Geometry check sheet. Reference: the model listing, model coordinates, mm. Face numbers are marked on the shaded views. A direction names the side the tool comes from. Coordinates: 2 decimals unless noted, no trailing zeros. Loops run counter-clockwise (first coordinate to the right, second up) from the corner with the lowest first, then second, coordinate; pieces in that order, holes last. Notation, with made-up numbers: M 52.25,23 L 89.25,23 A20 ccw 89.25,48 Z; hole C -3.5,57 d10. An arc over 180 degrees is marked long. One line per question, with ' | ' between items. Start each with the question number.
from build123d import *

# Parameters (mm, degrees)
M42_CLEARANCE_HOLE1_D                           = 47
M42_CLEARANCE_HOLE1_DEPTH                       = 4.5
SKETCH4_W                                       = 7
SKETCH4_H                                       = 4.5
CSK_FOR_M2_FLAT_HEAD_MACHINE_SCREW1_D           = 2.2
CSK_FOR_M2_FLAT_HEAD_MACHINE_SCREW1_DEPTH       = 6
CSK_FOR_M2_FLAT_HEAD_MACHINE_SCREW1_CSINK_D     = 4.4
CSK_FOR_M2_FLAT_HEAD_MACHINE_SCREW1_CSINK_ANGLE = 90
CBORE_FOR_M8_HEX_HEAD_BOLT1_D                   = 10
CBORE_FOR_M8_HEX_HEAD_BOLT1_DEPTH               = 6
CBORE_FOR_M8_HEX_HEAD_BOLT1_CBORE_D             = 11.2
CBORE_FOR_M8_HEX_HEAD_BOLT1_CBORE_DEPTH         = 1.2


with BuildPart() as part:
    # Sketch1 → Revolve1 (revolve)
    with BuildSketch(Plane(origin=(0, 0, 0), x_dir=(1, 0, 0), z_dir=(0, 1, 0))):
        Polygon((25.5, 0), (0, 0), (0, -6), (25.5, -6), (25.5, -5.5), (25, -5.5), (25, -0.5), (25.5, -0.5), align=None)
    revolve(axis=Axis((0, 0, 0), (0, 0, 1)))

    # M42 Clearance Hole1
    with Locations(Plane.XY.offset(6)):
        with Locations((0, 0)):
            Hole(M42_CLEARANCE_HOLE1_D / 2, depth=M42_CLEARANCE_HOLE1_DEPTH)

    # Sketch4 → Revolve2 (revolve)
    with BuildSketch(Plane(origin=(0, 0, 0), x_dir=(1, 0, 0), z_dir=(0, 1, 0))):
        with Locations((3.5, -3.75)):
            Rectangle(SKETCH4_W, SKETCH4_H)
    revolve(axis=Axis((0, 0, 1.5), (0, 0, 1)))

    # CSK for M2 Flat Head Machine Screw1
    with Locations(Plane(origin=(0, 0, 0), x_dir=(-1, 0, 0), z_dir=(0, 0, -1))):
        with Locations((-7.794228634, -4.5), (7.794228634, -4.5), (0, 9)):
            CounterSinkHole(CSK_FOR_M2_FLAT_HEAD_MACHINE_SCREW1_D / 2, CSK_FOR_M2_FLAT_HEAD_MACHINE_SCREW1_CSINK_D / 2, depth=CSK_FOR_M2_FLAT_HEAD_MACHINE_SCREW1_DEPTH, counter_sink_angle=CSK_FOR_M2_FLAT_HEAD_MACHINE_SCREW1_CSINK_ANGLE)

    # CBORE for M8 Hex Head Bolt1
    with Locations(Plane(origin=(0, 0, 0), x_dir=(-1, 0, 0), z_dir=(0, 0, -1))):
        with Locations((0, 0)):
            CounterBoreHole(CBORE_FOR_M8_HEX_HEAD_BOLT1_D / 2, CBORE_FOR_M8_HEX_HEAD_BOLT1_CBORE_D / 2, CBORE_FOR_M8_HEX_HEAD_BOLT1_CBORE_DEPTH, depth=CBORE_FOR_M8_HEX_HEAD_BOLT1_DEPTH)


solid = part.part
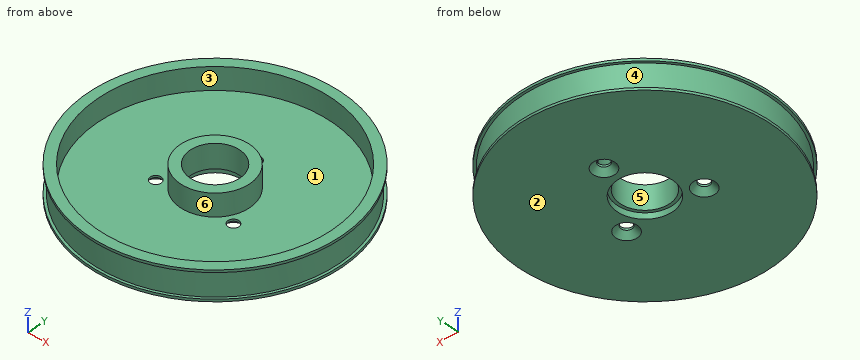
1. Sectioned sample at C-C (z = 2.35). Record the cut outline in (x, y), and give its area (3 significant figures).
2. Tool access check on the marked faces 5 and 6. Record the directions out of +Z, -Z, +X, -X, +Y, -Y that give a thin tool (end or side, any length) a straight path to the whole face; none if there is none.
3. Draft check along Z on the marked faces 1, 2, 3 and 4. Enter one of: +Z half, -Z half, draft (parallel to the pull), parting line (faces both ways), or undercut.
4. Sectioned sample at B-B (y = 0). Record the cut outline in (x, z), and give its area (3 significant figures).
5. Sectioned sample at D-D (y = -19). Record the cut outline in (x, z).
6. Depth check by flat-ended pin: pin 1 Ø1 at (x, y) = (-3, 7) entering from +Z; pin 2 Ø2.5 at (x, y) = (-7.79, -4.5) entering from -Z; pin 3 Ø3 at (x, y) = (0, 9) entering from -Z. Enter the tip coordinate at first touch or a pass-through.
7. Sectioned sample at A-A (x = 0). State how many separate pieces and enclosed holes the cut face has, and give its area (4 significant figures).
8. Thickness scan on line 1 (Y direction, x = 0, z = 1.3); line 2 (Y direction, x = -0.5, z = 0.4); line 3 (Z direction, x = 7.5, y = 18). Record the ranges inside material, lowest first.
Result:
1) outline: C 0,0 d50; C 0,0 d14; hole C 0,0 d47; hole C 0,0 d10 | area: 304 mm2
2) face 5: +Z, -Z | face 6: +Z
3) face 1: +Z half | face 2: -Z half | face 3: draft | face 4: undercut
4) outline: M -25.5,0 L -5.6,0 L -5.6,1.2 L -5,1.2 L -5,6 L -7,6 L -7,1.5 L -23.5,1.5 L -23.5,6 L -25.5,6 L -25.5,5.5 L -25,5.5 L -25,0.5 L -25.5,0.5 Z; M 5,1.2 L 5.6,1.2 L 5.6,0 L 25.5,0 L 25.5,0.5 L 25,0.5 L 25,5.5 L 25.5,5.5 L 25.5,6 L 23.5,6 L 23.5,1.5 L 7,1.5 L 7,6 L 5,6 Z | area: 91.1 mm2
5) outline: M -17.01,0 L 17.01,0 L 17.01,0.5 L 16.25,0.5 L 16.25,5.5 L 17.01,5.5 L 17.01,6 L 13.83,6 L 13.83,1.5 L -13.83,1.5 L -13.83,6 L -17.01,6 L -17.01,5.5 L -16.25,5.5 L -16.25,0.5 L -17.01,0.5 Z
6) pin 1: stops at z = 1.5 | pin 2: stops at z = 0.95 | pin 3: stops at z = 0.7
7) separate pieces: 3 | enclosed holes: 0 | area: 86.55 mm2
8) line 1: y = -25 to -5, 5 to 7.9, 10.1 to 25 | line 2: y = -25.5 to -5.58, 5.58 to 7.27, 10.73 to 25.5 | line 3: z = 0 to 1.5
